The figure shows three views and two pictorial views of one solid part (mm, origin at its lowest corner). Answer the questions. Give positions to 0.01 mm unless a question says otherwise; leave off trailing zeros. Write each loop counter-clockwise with the first axis right and the second up, starting at its lowest first coordinate (ties: lowest second). Pieces come first, ordered by that corner, then holes. Notation, with made-up numbers: (28.25, 22) -> (72.25, 22) arc R19 cw to (72.25, 55) -> close; hole circle Ø2 at (62.5, 50.25). An arc over 180 degrees is marked (long way). Write item = value, one per line. Start each with the question number.
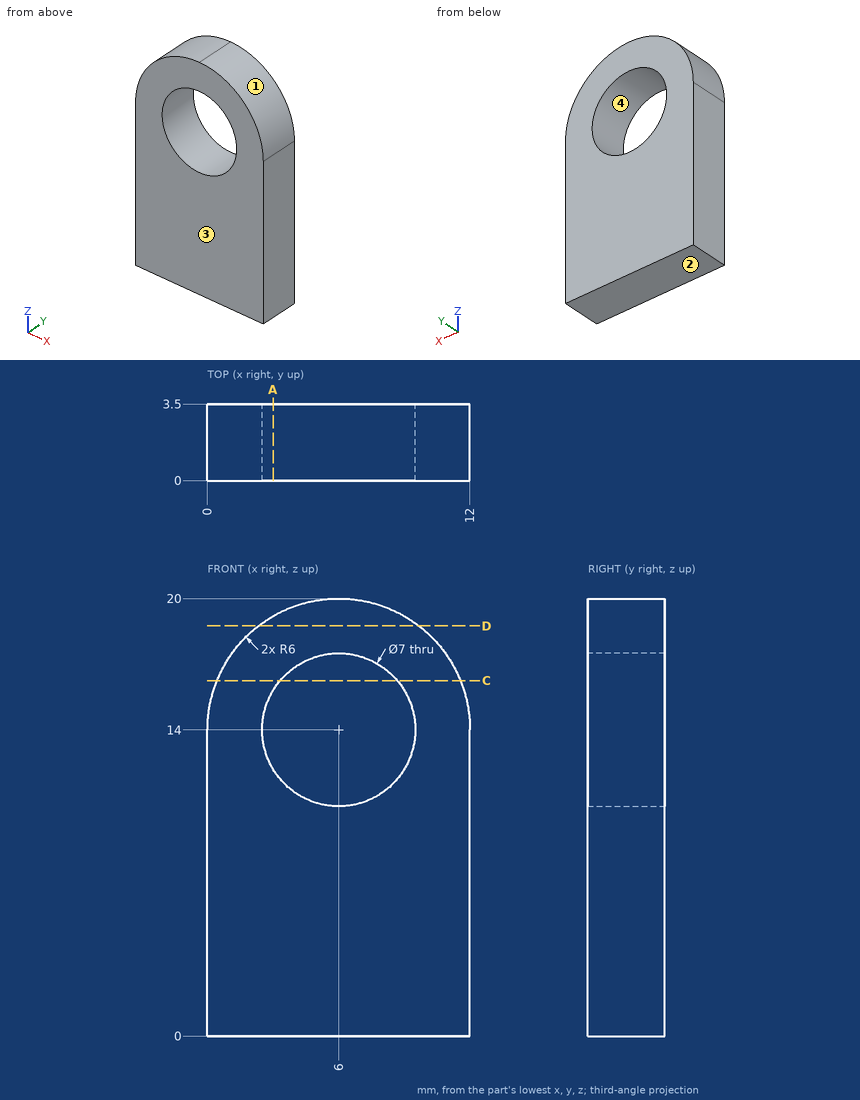
(1) A cutting plane is placed at D-D, the plane z = 18.75. Write down the section's boundary in (x, y), then the cut area to 3 significant figures.
(2) A cutting plane is placed at A-A, the plane x = 3. Write down the section's boundary in (y, z), then the cut area to 3 significant figures.
(3) This flat-tipped pin is pushed along its axis until it touches: pin 1 (1.5 mm diameter, centred on x = 9, z = 17.5, fed in from -Y). Where does it stop, or does it pass through?
(4) Find the intervals of material crossed by line 1 along X through (y, z) = (2.2, 14); line 2 along X through (y, z) = (1.3, 12.75); line 3 along Z through (x, y) = (6.5, 2.45), in increasing order.
(5) Determine the mould class of the marked faces 1, 2, 3 and 4 for opening direction Z: pulls with the +Z half, pulls with the -Z half, needs draft (parallel to the pull), parting line crosses it, or undercut.
(6) A cutting plane is placed at C-C, the plane z = 16.25. Write down the section's boundary in (x, y).
Results list:
q1.outline = (2.33, 0) -> (9.67, 0) -> (9.67, 3.5) -> (2.33, 3.5) -> close
q1.area = 25.7 mm²
q2.outline = (0, 0) -> (3.5, 0) -> (3.5, 12.2) -> (0, 12.2) -> close; (0, 15.8) -> (3.5, 15.8) -> (3.5, 19.2) -> (0, 19.2) -> close
q2.area = 54.6 mm²
q3.pin_1 = 0
q4.line_1 = 0 to 2.5, 9.5 to 12
q4.line_2 = 0 to 2.73, 9.27 to 12
q4.line_3 = 0 to 10.54, 17.46 to 19.98
q5.face_1 = pulls with the +Z half
q5.face_2 = pulls with the -Z half
q5.face_3 = needs draft
q5.face_4 = undercut
q6.outline = (0.44, 0) -> (3.32, 0) -> (3.32, 3.5) -> (0.44, 3.5) -> close; (8.68, 0) -> (11.56, 0) -> (11.56, 3.5) -> (8.68, 3.5) -> close
